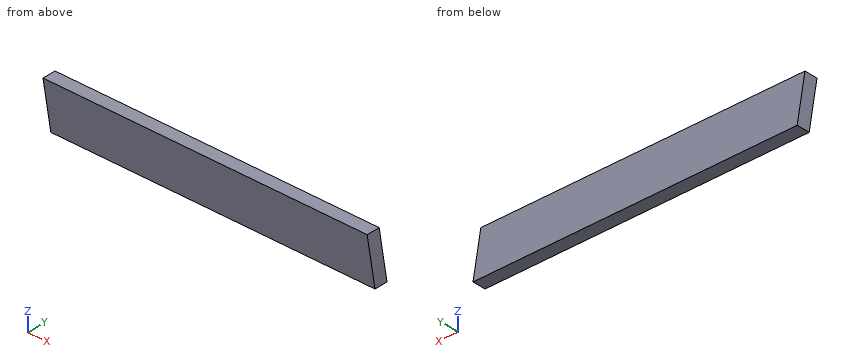
```python
from build123d import *

# Parameters (mm, degrees)
F0_W     = 476.25
F0_H     = 63.5
F1_DEPTH = 19.05
F3_DEPTH = 25.4
F5_DEPTH = 25.4


with BuildPart() as f1:
    # F0 (on Front) → F1 (new body)
    with BuildSketch(Plane.XZ):
        with Locations((-238.125, 31.75)):
            Rectangle(F0_W, F0_H)
    extrude(amount=F1_DEPTH)

    # F2 (on face) → F3 (cut)
    with BuildSketch(Plane.XZ.offset(19.05)):
        Polygon((-465.053237, 0), (-476.25, 63.5), (-476.25, 0), align=None)
    extrude(amount=-F3_DEPTH, mode=Mode.SUBTRACT)

    # F4 (on face) → F5 (cut)
    with BuildSketch(Plane.XZ.offset(19.05)):
        Polygon((-11.196763, 63.5), (0, 0), (0, 63.5), align=None)
    extrude(amount=-F5_DEPTH, mode=Mode.SUBTRACT)


solid = f1.part
```
Geometry: final body of the model. Coordinates: model frame, mm. Give positions to 0.01 mm unless a question says otherwise; leave off trailing zeros. Loops run counter-clockwise (first coordinate to the right, second up) from the corner with the lowest first, then second, coordinate; pieces in that order, holes last. Notation, with made-up numbers: (15.5, 21.5) - (62.5, 21.5) arc R23 cw to (62.5, 55.5) - close; hole circle Ø11 at (-12.75, 61). An arc over 180 degrees is marked (long way). Answer as CSV lines item,"result". Start each with the question number.
(1) Section query B-B (z = 46.5). Output: boundary loops of the cut face in (x, y).
(2) Ray query, line 1 along X through (y, z) = (-8, 50); line 2 along X through (y, z) = (-10.5, 11.5). Return the intervals inside material, ascending. Write a range as [from, to].
(3) Section query A-A (y = -8). Output: boundary loops of the cut face in (x, z), and give its area (3 significant figures).
(4) Pin query (flat end, axial travel): P1, Ø6, axis at y = -4.5, z = 55, coming from the -X side; P2, Ø3, axis at y = -9.5, z = 8, coming from the -X side; P3, Ø4, axis at y = -3, z = 32, coming from the -X side. Return the tip coordinate at first contact, or that it passes through.
Worked answers:
1,outline,"(-473.25, -19.05) - (-8.2, -19.05) - (-8.2, 0) - (-473.25, 0) - close"
2,line 1,"x = [-473.87, -8.82]"
2,line 2,"x = [-467.08, -2.03]"
3,outline,"(-476.25, 63.5) - (-465.05, 0) - (0, 0) - (-11.2, 63.5) - close"
3,area,"29,500 mm^2"
4,P1,"stops at x = -475.28"
4,P2,"stops at x = -466.73"
4,P3,"stops at x = -471.05"
